Autodesk Inventor part; units mm, degrees
ref_plane "Płaszczyzna konstrukcyjna1" through (0, 0.5, -17) normal (0, 0, -1) x (-1, 0, 0)
ref_plane "YZ Plane" through (0, 0, 0) normal (1, 0, 0) x (0, 1, 0)
ref_plane "XZ Plane" through (0, 0, 0) normal (0, 1, 0) x (-1, 0, 0)
sketch "Szkic1" plane through (0, 0, 0) normal (1, 0, 0) x (0, 1, 0)
  line L0 (0.5, 0) -> (6, 0)
  line L1 (22, 0) -> (22, -12) construction
  line L2 (22, -34) -> (18, -34) construction
  line L3 (0, -17) -> (11, -17) construction
  circle A0 centre (11, -17) radius 8
  line L4 (18, 0) -> (18, -1) construction
  line L5 (22, -12) -> (18, -8)
  line L6 (22, -12) -> (29.1229, -12) construction
  line L7 (22, -22) -> (18, -26)
  line L8 (22, -22) -> (32.7221, -22) construction
  line L9 (6, 0) -> (7, -1)
  line L10 (6, 0) -> (7.9702, 0) construction
  line L11 (7, -1) -> (17.5, -1)
  line L12 (6, 0) -> (22, 0) construction
  line L13 (18, -1.5) -> (18, -8)
  line L14 (22, -12) -> (22, -22)
  line L15 (22, -22) -> (22, -34) construction
  line L16 (18, -26) -> (18, -32.5)
  line L17 (18, -34) -> (6, -34) construction
  line L18 (17.5, -1) -> (18, -1.5)
  line L19 (17.3756, -0.6779) -> (19.849, -0.6779) construction
  line L20 (6, -34) -> (7, -33)
  line L21 (6, -34) -> (7.9702, -34) construction
  line L22 (17.5, -33) -> (18, -32.5)
  line L23 (7, -33) -> (17.5, -33)
  line L24 (6, -34) -> (0.5, -34)
  line L25 (18, -32.5) -> (18, -33)
  line L26 (0.5, 0) -> (0, -0.5)
  line L27 (0.5, -34) -> (0, -33.5)
  line L28 (0.5, -34) -> (0, -34) construction
  line L29 (0, -9.5) -> (0.5, -10)
  line L30 (0, -9.5) -> (3.9988, -9.5) construction
  line L31 (0.5, -10) -> (0.5, -24)
  line L32 (0, -24.5) -> (0.5, -24)
  line L33 (0, -34) -> (0, -24.5)
  line L34 (0, -9.5) -> (0, 0)
  line L35 (-6.5444, 0) -> (39.2665, 0)
  point P0 (17.3756, -33.3221)
  point P1 (3.25, 0)
  point P2 (0, -33.5)
  dimension "d0" = 22
  dimension "d1" = 34
  dimension "d3" = 16
  dimension "d5" = 135
  dimension "d6" = 135
  dimension "d7" = 10
  dimension "d8" = 12
  dimension "d9" = 45
  dimension "d12" = 45
  dimension "d13" = 0.5
  dimension "d15" = 0.5
  dimension "d16" = 45
  dimension "d17" = 10
  dimension "d19" = 11
  dimension "d20" = 0.5
  dimension "d21" = 18
  dimension "d22" = 135
  dimension "d23" = 1
  dimension "d24" = 6
extrude "Wyciągnięcie proste1" add sketch "Szkic1" along normal blind 30 contours L0 L9 L11 L18 L13 L5 L14 L7 L16 L22 L23 L20 L24 L27 L33 L32 L31 L29 L34 L26
chamfer "Faza1" distance 0.5 angle 45 2 edges at (30, 3, -17) (0, 3, -17)
ref_plane "Płaszczyzna konstrukcyjna1" through (0, 0.5, -17) normal (0, 0, -1) x (-1, 0, 0)
sketch "Szkic2" plane through (0, 0.5, -17) normal (0, 0, -1) x (-1, 0, 0)
  line L0 (-29.5, 18.5) -> (-0.5, 18.5)
  line L1 (-30, 21.5) -> (-30, 17.5)
  line L2 (-28.5, 18.5) -> (-28, 18.5)
  line L3 (-28, 18.5) -> (-28, 19.5)
  line L4 (-28, 19.5) -> (-28.5, 19.5)
  line L5 (-28.5, 19.5) -> (-28.5, 18.5)
  line L6 (0, 21.5) -> (-30, 21.5)
  line L7 (-15, 21.5) -> (-15, 18.5) construction
  line L8 (-1.5, 18.5) -> (-2, 18.5)
  line L9 (-2, 18.5) -> (-2, 19.5)
  line L10 (-2, 19.5) -> (-1.5, 19.5)
  line L11 (-1.5, 19.5) -> (-1.5, 18.5)
  line L12 (6, -0.5) -> (-36, -0.5)
  line L13 (-29.5, 2.5) -> (-29.5, 18.5)
  line L14 (-29.5, 10.5) -> (-0.5, 10.5) construction
  line L15 (-0.5, 18.5) -> (-0.5, 2.5)
  point P0 (0, -0.5)
  point P1 (-28.25, 18.5)
  point P2 (-1.75, 18.5)
  dimension "d31" = 0.5
  dimension "d32" = 1
  dimension "d33" = 1.5
revolve "Obrót1" cut sketch "Szkic2" angle 360 about axis through (29.5, 11, -17) along (-1, 0, 0)
sketch "Szkic3" plane through (0, 0, -33.5) normal (0, -1, 0) x (1, 0, 0)
  line L0 (24, 4.5) -> (6, 4.5) construction
  line L1 (6, 4.5) -> (6, 28.5) construction
  line L2 (6, 28.5) -> (24, 28.5) construction
  line L3 (24, 28.5) -> (24, 4.5) construction
  line L4 (0, 33.5) -> (30, 33.5)
  line L5 (0, 9) -> (0, 0)
  circle A0 centre (24, 4.5) radius 2
  circle A1 centre (6, 4.5) radius 2
  circle A2 centre (6, 28.5) radius 2
  circle A3 centre (24, 28.5) radius 2
  dimension "d35" = 18
  dimension "d36" = 24
  dimension "d37" = 5
  dimension "d38" = 6
  dimension "d39" = 4
  dimension "d40" = 4
  dimension "d41" = 4
  dimension "d42" = 4
extrude "Wyciągnięcie proste2" cut sketch "Szkic3" against normal blind 8
sketch "Szkic4" plane through (24, 8, -5) normal (0, -1, 0) x (1, 0, 0)
  circle A0 centre (0, 0) radius 2
  circle A1 centre (0, 0) radius 1.7
  circle A2 centre (-18, 0) radius 2
  circle A3 centre (-18, 0) radius 1.7
  circle A4 centre (-18, -24) radius 2
  circle A5 centre (-18, -24) radius 1.7
  circle A6 centre (0, -24) radius 2
  circle A7 centre (0, -24) radius 1.7
  point P0 (-24, 5)
  dimension "d45" = 3.4
  dimension "d46" = 3.4
  dimension "d47" = 3.4
  dimension "d48" = 3.4
extrude "Wyciągnięcie proste3" cut sketch "Szkic4" against normal up to surface (10 mm away) contours A1 | A3 | A5 | A7
chamfer "Faza2" distance 0.25 angle 45 8 edges at (22.3, 18, -29) (4.3, 18, -29) (4.3, 18, -5) (22.3, 18, -5) (22, 0, -5) (4, 0, -5) (22, 0, -29) (4, 0, -29)
fillet "Zaokrąglenie1" radius 0.25 42 edges at (0, 3.25, -34) (0, 0.25, -33.75) (0, 0, -29) (0, 0.25, -24.25) (0, 0.5, -17) (0, 0.25, -9.75) (0, 0, -5) (0, 0.25, -0.25) (0, 3.25, 0) (0, 6.5, -0.5) (0, 12.25, -1) (0, 17.75, -1.25) (0, 18, -4.75) (0, 20, -10) (0, 22, -17) (0, 20, -24) (0, 18, -29.25) (0, 17.75, -32.75) (0, 12.25, -33) (0, 6.5, -33.5) (30, 3.25, -34) (30, 6.5, -33.5) (30, 12.25, -33) (30, 17.75, -32.75) (30, 18, -29.25) (30, 20, -24) (30, 22, -17) (30, 20, -10) (30, 18, -4.75) (30, 17.75, -1.25) (30, 12.25, -1) (30, 6.5, -0.5) (30, 3.25, 0) (30, 0.25, -0.25) (30, 0, -5) (30, 0.25, -9.75) (30, 0.5, -17) (30, 0.25, -24.25) (30, 0, -29) (30, 0.25, -33.75) (15, 22, -22) (15, 22, -12)
chamfer "Faza3" distance 0.05 angle 45 4 edges at (2, 3, -17) (1.5, 3, -17) (28, 3, -17) (28.5, 3, -17)
properties part number "SC8UU body"
Here's how the part is built. I have some questions about the finished solid (model axes, mm). A direction names the side the tool comes from. Give positions to 0.01 mm unless a question says otherwise; leave off trailing zeros. Order: outer loops, then holes, each group sorted by start corner. A loop starts at its lowest first (then second) coordinate and runs counter-clockwise, first axis right, second up. Notation, with made-up numbers: (89.5, 42) -> (140.5, 42) arc R30 cw to (140.5, 68) -> close; hole circle Ø8 at (37, 88.25). An arc over 180 degrees is marked (long way). One line per item, written item: value. Start each with the question number.
1. Imagine slicing it at B-B, the plane x = 9.25. List the corners of the cut face in (y, z) for me.
2. Imagine slicing it at A-A, the plane z = -29. Count the separate pieces of the cut face and the enclosed holes in it, plus the area to 3 significant figures.
3. We'd pull the mould along X, two halves only. Please class faces 3 (the face through (0.075, 6.494, -33.405)), 4 (the face through (25.57, 12.81, -29.65)), 5 (the face through (15, 12, -1)): released by +X, released by -X, zero draft, split by the parting line, or undercut.
4. I need wall thicknesses on probe 1 along Z at (x, y) = (22.5, 3.75); probe 2 along Z at (x, y) = (14.5, 11); probe 3 along Y at (x, z) = (28.9, -17). Which ranges of each line are inside material? Lowest first, please. Write a range as from..to.
5. For faces 1 (the face through (29.02, 9.27, -9.19)), 2 (the face through (28.254, 19.314, -20.447)), which set-ups out of +Z, -Z, +X, -X, +Y, -Y let a thin tool reach every point of the face, with its end or its side?
6. Will these pins go through, and if not, where does the flat tip stop? pin 1 Ø9.5 at (y, z) = (11, -17) entering from +X; pin 2 Ø5 at (x, z) = (22, -27.5) entering from +Y; pin 3 Ø10 at (x, z) = (24, -30.5) entering from +Y; pin 4 Ø5 at (x, y) = (8.5, 17.5) entering from +Z.
Values follow:
1. outline: (0, -33.5) -> (0.5, -34) -> (6, -34) -> (7, -33) -> (17.5, -33) -> (18, -32.5) -> (18, -26) -> (21.93, -22.07) arc R0.25 ccw to (22, -21.9) -> (22, -12.1) arc R0.25 ccw to (21.93, -11.93) -> (18, -8) -> (18, -1.5) -> (17.5, -1) -> (7, -1) -> (6, 0) -> (0.5, 0) -> (0, -0.5) -> (0, -9.5) -> (0.5, -10) -> (0.5, -24) -> (0, -24.5) -> close; hole circle Ø16 at (11, -17)
2. separate pieces: 3
2. enclosed holes: 0
2. area: 408 mm2
3. face 3: released by -X
3. face 4: undercut
3. face 5: zero draft
4. probe 1: z = -34..-30.32, -27.68..-20.38, -13.62..-6.32, -3.68..0
4. probe 2: z = -33..-25, -9..-1
4. probe 3: y = 0.5..3, 19..22
5. face 1: +X, -X
5. face 2: none
6. pin 1: passes through
6. pin 2: stops at y = 19
6. pin 3: stops at y = 18.5
6. pin 4: stops at z = -1
